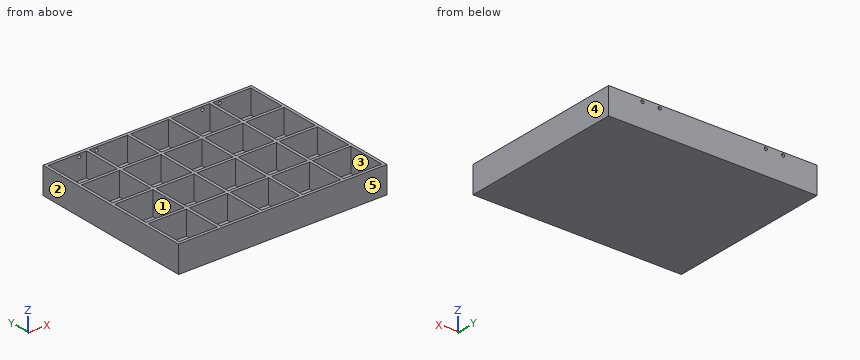
Autodesk Inventor part; units mm, degrees
ref_plane "YZ Plane" through (0, 0, 0) normal (1, 0, 0) x (0, 1, 0)
ref_plane "XZ Plane" through (0, 0, 0) normal (0, 1, 0) x (-1, 0, 0)
ref_plane "XY Plane" through (0, 0, 0) normal (0, 0, 1) x (1, 0, 0)
sketch "Sketch1" plane through (0, 0, 0) normal (0, 0, 1) x (1, 0, 0)
  line L0 (-109, -87.5) -> (109, -87.5)
  line L1 (109, -87.5) -> (109, 87.5)
  line L2 (109, 87.5) -> (-109, 87.5)
  line L3 (-109, 87.5) -> (-109, -87.5)
  line L4 (-109, -87.5) -> (109, 87.5) construction
  line L5 (109, -87.5) -> (-109, 87.5) construction
  point P0 (0, 0)
  dimension "d0" = 218
  dimension "d1" = 175
extrude "Extrusion1" add sketch "Sketch1" along normal blind 28
sketch "Sketch2" plane through (0, 0, 28) normal (0, 0, 1) x (1, 0, 0)
  line L0 (-106, 84.5) -> (-66, 84.5)
  line L1 (-66, 84.5) -> (-66, 44.5)
  line L2 (-66, 44.5) -> (-106, 44.5)
  line L3 (-106, 44.5) -> (-106, 84.5)
  line L4 (-106, 84.5) -> (-66, 44.5) construction
  line L5 (-66, 84.5) -> (-106, 44.5) construction
  line L6 (109, 87.5) -> (-109, 87.5)
  line L7 (-109, 87.5) -> (-109, -87.5)
  line L8 (-63, 84.5) -> (-23, 84.5)
  line L9 (-23, 84.5) -> (-23, 44.5)
  line L10 (-23, 44.5) -> (-63, 44.5)
  line L11 (-63, 44.5) -> (-63, 84.5)
  line L12 (-63, 84.5) -> (-23, 44.5) construction
  line L13 (-23, 84.5) -> (-63, 44.5) construction
  line L14 (-20, 84.5) -> (20, 84.5)
  line L15 (20, 84.5) -> (20, 44.5)
  line L16 (20, 44.5) -> (-20, 44.5)
  line L17 (-20, 44.5) -> (-20, 84.5)
  line L18 (-20, 84.5) -> (20, 44.5) construction
  line L19 (20, 84.5) -> (-20, 44.5) construction
  line L20 (23, 84.5) -> (63, 84.5)
  line L21 (63, 84.5) -> (63, 44.5)
  line L22 (63, 44.5) -> (23, 44.5)
  line L23 (23, 44.5) -> (23, 84.5)
  line L24 (23, 84.5) -> (63, 44.5) construction
  line L25 (63, 84.5) -> (23, 44.5) construction
  line L26 (66, 84.5) -> (106, 84.5)
  line L27 (106, 84.5) -> (106, 44.5)
  line L28 (106, 44.5) -> (66, 44.5)
  line L29 (66, 44.5) -> (66, 84.5)
  line L30 (66, 84.5) -> (106, 44.5) construction
  line L31 (106, 84.5) -> (66, 44.5) construction
  line L32 (-106, 41.5) -> (-66, 41.5)
  line L33 (-66, 41.5) -> (-66, 1.5)
  line L34 (-66, 1.5) -> (-106, 1.5)
  line L35 (-106, 1.5) -> (-106, 41.5)
  line L36 (-106, 41.5) -> (-66, 1.5) construction
  line L37 (-66, 41.5) -> (-106, 1.5) construction
  line L38 (-63, 41.5) -> (-23, 41.5)
  line L39 (-23, 41.5) -> (-23, 1.5)
  line L40 (-23, 1.5) -> (-63, 1.5)
  line L41 (-63, 1.5) -> (-63, 41.5)
  line L42 (-63, 41.5) -> (-23, 1.5) construction
  line L43 (-23, 41.5) -> (-63, 1.5) construction
  line L44 (-20, 41.5) -> (20, 41.5)
  line L45 (20, 41.5) -> (20, 1.5)
  line L46 (20, 1.5) -> (-20, 1.5)
  line L47 (-20, 1.5) -> (-20, 41.5)
  line L48 (-20, 41.5) -> (20, 1.5) construction
  line L49 (20, 41.5) -> (-20, 1.5) construction
  line L50 (23, 41.5) -> (63, 41.5)
  line L51 (63, 41.5) -> (63, 1.5)
  line L52 (63, 1.5) -> (23, 1.5)
  line L53 (23, 1.5) -> (23, 41.5)
  line L54 (23, 41.5) -> (63, 1.5) construction
  line L55 (63, 41.5) -> (23, 1.5) construction
  line L56 (66, 41.5) -> (106, 41.5)
  line L57 (106, 41.5) -> (106, 1.5)
  line L58 (106, 1.5) -> (66, 1.5)
  line L59 (66, 1.5) -> (66, 41.5)
  line L60 (66, 41.5) -> (106, 1.5) construction
  line L61 (106, 41.5) -> (66, 1.5) construction
  line L62 (-106, -1.5) -> (-66, -1.5)
  line L63 (-66, -1.5) -> (-66, -41.5)
  line L64 (-66, -41.5) -> (-106, -41.5)
  line L65 (-106, -41.5) -> (-106, -1.5)
  line L66 (-106, -1.5) -> (-66, -41.5) construction
  line L67 (-66, -1.5) -> (-106, -41.5) construction
  line L68 (-63, -1.5) -> (-23, -1.5)
  line L69 (-23, -1.5) -> (-23, -41.5)
  line L70 (-23, -41.5) -> (-63, -41.5)
  line L71 (-63, -41.5) -> (-63, -1.5)
  line L72 (-63, -1.5) -> (-23, -41.5) construction
  line L73 (-23, -1.5) -> (-63, -41.5) construction
  line L74 (-20, -1.5) -> (20, -1.5)
  line L75 (20, -1.5) -> (20, -41.5)
  line L76 (20, -41.5) -> (-20, -41.5)
  line L77 (-20, -41.5) -> (-20, -1.5)
  line L78 (-20, -1.5) -> (20, -41.5) construction
  line L79 (20, -1.5) -> (-20, -41.5) construction
  line L80 (23, -1.5) -> (63, -1.5)
  line L81 (63, -1.5) -> (63, -41.5)
  line L82 (63, -41.5) -> (23, -41.5)
  line L83 (23, -41.5) -> (23, -1.5)
  line L84 (23, -1.5) -> (63, -41.5) construction
  line L85 (63, -1.5) -> (23, -41.5) construction
  line L86 (66, -1.5) -> (106, -1.5)
  line L87 (106, -1.5) -> (106, -41.5)
  line L88 (106, -41.5) -> (66, -41.5)
  line L89 (66, -41.5) -> (66, -1.5)
  line L90 (66, -1.5) -> (106, -41.5) construction
  line L91 (106, -1.5) -> (66, -41.5) construction
  line L92 (-106, -44.5) -> (-66, -44.5)
  line L93 (-66, -44.5) -> (-66, -84.5)
  line L94 (-66, -84.5) -> (-106, -84.5)
  line L95 (-106, -84.5) -> (-106, -44.5)
  line L96 (-106, -44.5) -> (-66, -84.5) construction
  line L97 (-66, -44.5) -> (-106, -84.5) construction
  line L98 (-63, -44.5) -> (-23, -44.5)
  line L99 (-23, -44.5) -> (-23, -84.5)
  line L100 (-23, -84.5) -> (-63, -84.5)
  line L101 (-63, -84.5) -> (-63, -44.5)
  line L102 (-63, -44.5) -> (-23, -84.5) construction
  line L103 (-23, -44.5) -> (-63, -84.5) construction
  line L104 (-20, -44.5) -> (20, -44.5)
  line L105 (20, -44.5) -> (20, -84.5)
  line L106 (20, -84.5) -> (-20, -84.5)
  line L107 (-20, -84.5) -> (-20, -44.5)
  line L108 (-20, -44.5) -> (20, -84.5) construction
  line L109 (20, -44.5) -> (-20, -84.5) construction
  line L110 (23, -44.5) -> (63, -44.5)
  line L111 (63, -44.5) -> (63, -84.5)
  line L112 (63, -84.5) -> (23, -84.5)
  line L113 (23, -84.5) -> (23, -44.5)
  line L114 (23, -44.5) -> (63, -84.5) construction
  line L115 (63, -44.5) -> (23, -84.5) construction
  line L116 (66, -44.5) -> (106, -44.5)
  line L117 (106, -44.5) -> (106, -84.5)
  line L118 (106, -84.5) -> (66, -84.5)
  line L119 (66, -84.5) -> (66, -44.5)
  line L120 (66, -44.5) -> (106, -84.5) construction
  line L121 (106, -44.5) -> (66, -84.5) construction
  point P0 (0, 0)
  point P1 (-86, 64.5)
  point P2 (-43, 64.5)
  point P3 (0, 64.5)
  point P4 (43, 64.5)
  point P5 (86, 64.5)
  point P6 (-86, 21.5)
  point P7 (-43, 21.5)
  point P8 (0, 21.5)
  point P9 (43, 21.5)
  point P10 (86, 21.5)
  point P11 (-86, -21.5)
  point P12 (-43, -21.5)
  point P13 (0, -21.5)
  point P14 (43, -21.5)
  point P15 (86, -21.5)
  point P16 (-86, -64.5)
  point P17 (-43, -64.5)
  point P18 (0, -64.5)
  point P19 (43, -64.5)
  point P20 (86, -64.5)
  dimension "d4" = 40
  dimension "d5" = 3
  dimension "d6" = 3
  dimension "d7" = 40
  dimension "d10" = 43
  dimension "d13" = 43
extrude "Extrusion2" cut sketch "Sketch2" against normal blind 25
sketch "Sketch3" plane through (-109, 87.5, 0) normal (0, 1, 0) x (1, 0, 0)
  line L0 (46, -28) -> (46, -3) construction
  line L1 (43, -28) -> (43, -3) construction
  line L2 (43, -28) -> (43, -3)
  line L3 (43, -25) -> (46, -25) construction
  line L4 (46, -28) -> (46, -3)
  line L5 (218, -28) -> (0, -28)
  circle A0 centre (53.5, -25) radius 1.65
  circle A1 centre (35.5, -25) radius 1.65
  line L6 (172, -28) -> (172, -3) construction
  line L7 (175, -28) -> (175, -3) construction
  line L8 (172, -28) -> (172, -3)
  line L9 (172, -25) -> (175, -25) construction
  circle A2 centre (182.5, -25) radius 1.65
  circle A3 centre (164.5, -25) radius 1.65
  point P0 (109, 0)
  point P1 (44.5, -25)
  point P2 (173.5, -25)
  dimension "d20" = 3
  dimension "d21" = 3.3
  dimension "d22" = 9
  dimension "d23" = 3.3
  dimension "d24" = 9
  dimension "d25" = 3.3
  dimension "d27" = 9
  dimension "d30" = 3
  dimension "d31" = 3.3
  dimension "d32" = 9
extrude "Extrusion3" cut sketch "Sketch3" against normal blind 10
equation "\"d0\" = box_length"
equation "\"d1\" = box_width"
equation "\"d2\" = hole_height + wall"
equation "\"d4\" = hole"
equation "\"d5\" = wall"
equation "\"d6\" = wall"
equation "\"d7\" = hole"
equation "\"d10\" = hole + wall"
equation "\"d13\" = hole + wall"
equation "\"d16\" = hole_height"
equation "\"d23\" = d21"
equation "\"d25\" = d21"
equation "\"d31\" = d25"
equation "\"hole\" = 40"
equation "\"wall\" = 3"
equation "\"hole_height\" = 25"
properties part number "RatPelletBox_v02"
Geometry check sheet. Reference: the model listing, model coordinates, mm. Face numbers are marked on the shaded views. A direction names the side the tool comes from. Round coordinates to 2 decimals unless told otherwise and drop trailing zeros. Loops run counter-clockwise (first coordinate to the right, second up) from the corner with the lowest first, then second, coordinate; pieces in that order, holes last. Notation, with made-up numbers: (-26.75, 86) - (4.25, 86) arc R26 ccw to (4.25, 103) - close; hole circle Ø6 at (71, -19.5). An arc over 180 degrees is marked (long way). Write item = value, one per line. Start each with the question number.
1. Set-up check for the marked faces 1 and 2: record each of +Z, -Z, +X, -X, +Y, -Y from which the full face is reachable in a straight line by a thin tool's end or side.
2. Section check A-A on y = -49. Enter the section's corners in (x, z).
3. Section check C-C on z = 8.25. Give the number of separate pieces and of enclosed holes in the cut face, then the cut area to 3 significant figures.
4. Depth check by flat-ended pin: pin 1 (20 mm diameter, centred on x = 79, y = -19.5, fed in from +Z). Enter the tip coordinate at first touch or a pass-through.
5. Section check B-B on x = 68.5. Enter the section's corners in (y, z).
6. Mould release check, pull along Y, two halves, no side actions. Record for the marked faces 3, 4 and 5: released by +Y, released by -Y, zero draft, split by the parting line, or undercut.
7. Thickness scan on line 1 (X direction, y = 49, z = 17.75); line 2 (X direction, y = 85.95, z = 25); line 3 (Y direction, x = 80.5, z = 13.5). Record the ranges inside material, lowest first.
Working result:
q1.face_1 = +Z
q1.face_2 = +Z, -Z, -X, +Y, -Y
q2.outline = (-109, 0) - (109, 0) - (109, 28) - (106, 28) - (106, 3) - (66, 3) - (66, 28) - (63, 28) - (63, 3) - (23, 3) - (23, 28) - (20, 28) - (20, 3) - (-20, 3) - (-20, 28) - (-23, 28) - (-23, 3) - (-63, 3) - (-63, 28) - (-66, 28) - (-66, 3) - (-106, 3) - (-106, 28) - (-109, 28) - close
q3.separate_pieces = 1
q3.enclosed_holes = 20
q3.area = 6,150 mm^2
q4.pin_1 = 3
q5.outline = (-87.5, 0) - (87.5, 0) - (87.5, 28) - (84.5, 28) - (84.5, 3) - (44.5, 3) - (44.5, 28) - (41.5, 28) - (41.5, 3) - (1.5, 3) - (1.5, 28) - (-1.5, 28) - (-1.5, 3) - (-41.5, 3) - (-41.5, 28) - (-44.5, 28) - (-44.5, 3) - (-84.5, 3) - (-84.5, 28) - (-87.5, 28) - close
q6.face_3 = undercut
q6.face_4 = zero draft
q6.face_5 = released by -Y
q7.line_1 = -109 to -106, -66 to -63, -23 to -20, 20 to 23, 63 to 66, 106 to 109
q7.line_2 = -109 to -75.15, -71.85 to -57.15, -53.85 to 53.85, 57.15 to 71.85, 75.15 to 109
q7.line_3 = -87.5 to -84.5, -44.5 to -41.5, -1.5 to 1.5, 41.5 to 44.5, 84.5 to 87.5
